Read the model definition and answer for the solid it produces. Units are mm, in the model's axes. Face numbers are marked on the shaded views. Give positions to 0.01 mm unless a question says otherwise; leave off trailing zeros. Order: outer loops, then holes, each group sorted by start corner. A loop starts at its lowest first (then second) coordinate and runs counter-clockwise, first axis right, second up. Notation, with made-up numbers: (70, 67.5) - (95, 67.5) arc R21 cw to (95, 94.5) - close; hole circle Ø5 at (85.25, 72.25). An arc over 180 degrees is marked (long way). Write each question's results on one line, items separated by ' | '. Start each with the question number.
Q1. Find the intervals of material crossed by line 1 along Y through (x, z) = (0, 1.6); line 2 along X through (y, z) = (13, 1.8); line 3 along X through (y, z) = (-15.5, 0.3), in increasing order. Write a range as from..to.
Q2. Find section A-A on y = 0. Give the vertices of the cut face in (x, z), and give its area (3 significant figures).
Q3. Find section C-C on y = -6. Give the vertices of the cut face in (x, z), and give its area (3 significant figures).
Q4. Find section D-D on x = 11.5. Give the vertices of the cut face in (y, z), and give its area (3 significant figures).
Q5. For a pull along X with two mould halves and no side action, classify the marked faces 1, 2 and 3 as +X half, -X half, draft (parallel to the pull), parting line (faces both ways), or undercut.
Q6. A flat-ended cylindrical pin translates along its axis: P1, Ø1.5, axis at x = -7.5, y = -17.5, coming from the -Z side. Find the tip coordinate at first contact, or state that the pin passes through.
from build123d import *

# Parameters (mm, degrees)
SKETCH1_R           = 25
SKETCH1_R_2         = 10
BOSS_EXTRUDE1_DEPTH = 5
CIRPATTERN1_COUNT   = 4
CIRPATTERN2_COUNT   = 4


with BuildPart() as part:
    # Sketch1 → Boss-Extrude1 (new body)
    with BuildSketch(Plane.XY):
        Circle(SKETCH1_R)
        Circle(SKETCH1_R_2, mode=Mode.SUBTRACT)
    extrude(amount=BOSS_EXTRUDE1_DEPTH)

    # Sketch4 → M3 Clearance Hole1 (revolve, cut)
    with BuildSketch(Plane(origin=(0, 12.5, 5), x_dir=(0, -1, 0), z_dir=(1, 0, 0))):
        Polygon((0, 0), (0, 8.521463052), (1.7, 7.5), (1.7, 0), align=None)
    m3_clearance_hole1 = revolve(axis=Axis((0, 12.5, 11.35), (0, 0, -1)), mode=Mode.SUBTRACT)

    # CirPattern1: M3 Clearance Hole1 ×4 about axis
    cirpattern1_axis = Axis((0, 0, 0), (0, 0, 1))
    for i in range(1, CIRPATTERN1_COUNT):
        add(m3_clearance_hole1.rotate(cirpattern1_axis, i * 360 / CIRPATTERN1_COUNT), mode=Mode.SUBTRACT)

    # Sketch6 → M3 Clearance Hole2 (revolve, cut)
    with BuildSketch(Plane(origin=(14.142135624, 14.142135624, 5), x_dir=(0, -1, 0), z_dir=(1, 0, 0))):
        Polygon((0, 0), (0, 8.521463052), (1.7, 7.5), (1.7, 0), align=None)
    m3_clearance_hole2 = revolve(axis=Axis((14.142135624, 14.142135624, 11.35), (0, 0, -1)), mode=Mode.SUBTRACT)

    # CirPattern2: M3 Clearance Hole2 ×4 about axis
    cirpattern2_axis = Axis((0, 0, 0), (0, 0, 1))
    for i in range(1, CIRPATTERN2_COUNT):
        add(m3_clearance_hole2.rotate(cirpattern2_axis, i * 360 / CIRPATTERN2_COUNT), mode=Mode.SUBTRACT)


solid = part.part
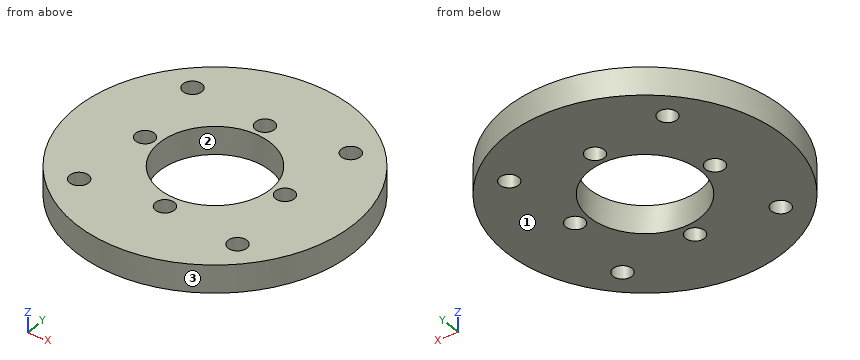
Working result:
1) line 1: -25..-14.2, -10.8..-10, 10..10.8, 14.2..25 | line 2: -21.35..-15.4, -12.88..-1.62, 1.62..12.88, 15.4..21.35 | line 3: -19.62..-15.16, -13.12..13.12, 15.16..19.62
2) outline: (-25, 0) - (-14.2, 0) - (-14.2, 5) - (-25, 5) - close; (-10.8, 0) - (-10, 0) - (-10, 5) - (-10.8, 5) - close; (10, 0) - (10.8, 0) - (10.8, 5) - (10, 5) - close; (14.2, 0) - (25, 0) - (25, 5) - (14.2, 5) - close | area: 116 mm²
3) outline: (-24.27, 0) - (-8, 0) - (-8, 5) - (-24.27, 5) - close; (8, 0) - (24.27, 0) - (24.27, 5) - (8, 5) - close | area: 163 mm²
4) outline: (-22.2, 0) - (-1.37, 0) - (-1.37, 5) - (-22.2, 5) - close; (1.37, 0) - (22.2, 0) - (22.2, 5) - (1.37, 5) - close | area: 208 mm²
5) face 1: draft | face 2: undercut | face 3: parting line
6) P1: z = 0
